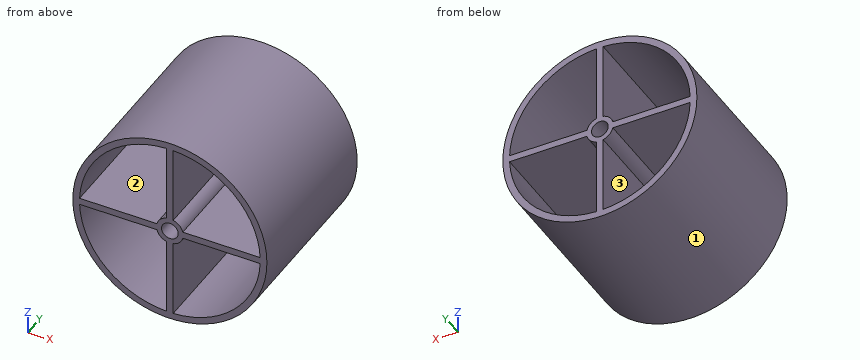
Autodesk Inventor part; units mm, degrees
ref_plane "YZ Plane" through (0, 0, 0) normal (1, 0, 0) x (0, 1, 0)
ref_plane "XZ Plane" through (0, 0, 0) normal (0, 1, 0) x (-1, 0, 0)
ref_plane "XY Plane" through (0, 0, 0) normal (0, 0, 1) x (1, 0, 0)
sketch "Boceto1" plane through (0, 0, 0) normal (0, 1, 0) x (-1, 0, 0)
  circle A0 centre (0, 0) radius 29
  dimension "d0" = 58
extrude "Extrusión1" add sketch "Boceto1" along normal blind 50
shell "Vaciado1" thickness 2 removed faces 2 at (2.104, 0, -7.1206) at (2.104, 50, -7.1206)
sketch "Boceto2" plane through (0, 0, 0) normal (0, -1, 0) x (1, 0, 0)
  line L0 (1, 28.5) -> (-1, 28.5)
  line L1 (-1, -28.5) -> (1, -28.5)
  line L2 (-28.5, 1) -> (-28.5, -1)
  line L3 (28.5, -1) -> (28.5, 1)
  line L4 (-19.4454, 20.8597) -> (-20.8597, 19.4454)
  line L5 (19.4454, -20.8597) -> (20.8597, -19.4454)
  line L6 (-64.7852, 95.7171) -> (-23.0659, 56.8262) construction
  line L7 (-20.8597, -19.4454) -> (-19.4454, -20.8597)
  line L8 (20.8597, 19.4454) -> (19.4454, 20.8597)
  arc A0 (-1, 3.873) -> (-2.0315, 3.4457) centre (0, 0) ccw
  line L9 (-1, 28.5) -> (-1, 3.873)
  line L10 (-3.873, 1) -> (-28.5, 1)
  line L11 (-28.5, -1) -> (-3.873, -1)
  line L12 (3.873, -1) -> (28.5, -1)
  line L13 (28.5, 1) -> (3.873, 1)
  line L14 (-1, -3.873) -> (-1, -28.5)
  line L15 (1, -28.5) -> (1, -3.873)
  line L16 (1, 3.873) -> (1, 28.5)
  arc A1 (3.873, 1) -> (1, 3.873) centre (0, 0) ccw
  arc A2 (1, -3.873) -> (3.873, -1) centre (0, 0) ccw
  arc A3 (1, -3.873) -> (3.873, -1) centre (0, 0) ccw
  arc A4 (-3.873, -1) -> (-1, -3.873) centre (0, 0) ccw
  arc A5 (-3.873, -1) -> (-1, -3.873) centre (0, 0) ccw
  arc A6 (-3.4457, 2.0315) -> (-3.873, 1) centre (0, 0) ccw
  arc A7 (3.873, 1) -> (1, 3.873) centre (0, 0) ccw
  arc A8 (-1, 3.873) -> (-3.873, 1) centre (0, 0) ccw
  circle A9 centre (0, 0) radius 2.5
  dimension "d4" = 2
  dimension "d5" = 57
  dimension "d6" = 57
  dimension "d7" = 2
  dimension "d12" = 2
  dimension "d13" = 57
  dimension "d14" = 57
  dimension "d15" = 2
  dimension "d17" = 5
extrude "Extrusión2" add sketch "Boceto2" against normal blind 50
properties part number "Tambor"
Read the model definition and answer for the solid it produces. Units are mm, in the model's axes. Face numbers are marked on the shaded views. Give positions to 0.01 mm unless a question says otherwise; leave off trailing zeros. Write each loop counter-clockwise with the first axis right and the second up, starting at its lowest first coordinate (ties: lowest second). Pieces come first, ordered by that corner, then holes. Notation, with made-up numbers: (17, 66) - (76, 66) arc R15 ccw to (76, 82) - close; hole circle Ø9 at (-11, -1). An arc over 180 degrees is marked (long way). Return JSON: item names as keys, results as strings.
Q1. A cutting plane is placed at C-C, the plane y = 41. Determine the outline of the cut face in (x, z), and give its area (3 significant figures).
Reply:
{"outline": "circle Ø58 at (0, 0); hole (-26.98, -1) arc R27 ccw to (-1, -26.98) - (-1, -3.87) arc R4 cw to (-3.87, -1) - close; hole (-26.98, 1) - (-3.87, 1) arc R4 cw to (-3.45, 2.03) arc R4 cw to (-2.03, 3.45) arc R4 cw to (-1, 3.87) - (-1, 26.98) arc R27 ccw to start; hole circle Ø5 at (0, 0); hole (1, -26.98) arc R27 ccw to (26.98, -1) - (3.87, -1) arc R4 cw to (1, -3.87) - close; hole (1, 3.87) arc R4 cw to (3.87, 1) - (26.98, 1) arc R27 ccw to (1, 26.98) - close", "area": "567 mm²"}
Q2. A cutting plane is placed at A-A, the plane z = 0. Determine the outline of the cut face in (x, y).
Reply:
{"outline": "(-29, 0) - (-2.5, 0) - (-2.5, 50) - (-29, 50) - close; (2.5, 0) - (29, 0) - (29, 50) - (2.5, 50) - close"}
Q3. A cutting plane is placed at B-B, the plane x = 0. Determine the outline of the cut face in (y, z).
Reply:
{"outline": "(0, -29) - (50, -29) - (50, -2.5) - (0, -2.5) - close; (0, 2.5) - (50, 2.5) - (50, 29) - (0, 29) - close"}
Q4. Consider line 1 along Z through (x, y) = (0, 25); line 2 along X through (y, z) = (21, 11); line 3 along X through (y, z) = (38, -14.5). Determine where each line is inside the solid, lowest interval first. Write a range as [from, to].
Reply:
{"line 1": "[-29, -2.5], [2.5, 29]", "line 2": "[-26.83, -24.66], [-1, 1], [24.66, 26.83]", "line 3": "[-25.11, -22.78], [-1, 1], [22.78, 25.11]"}
Q5. For a pull along Z with two mould halves and no side action, classify the marked faces 1, 2 and 3 as released by +Z, released by -Z, zero draft, split by the parting line, or undercut.
Reply:
{"face 1": "split by the parting line", "face 2": "undercut", "face 3": "undercut"}
Q6. A cutting plane is placed at D-D, the plane z = 13. Determine the outline of the cut face in (x, y), and give its area (3 significant figures).
Reply:
{"outline": "(-25.92, 0) - (-23.66, 0) - (-23.66, 50) - (-25.92, 50) - close; (-1, 0) - (1, 0) - (1, 50) - (-1, 50) - close; (23.66, 0) - (25.92, 0) - (25.92, 50) - (23.66, 50) - close", "area": "326 mm²"}
Q7. Given P1, Ø11.5, axis at x = 12.5, y = 24, coming from the -Z side; P2, Ø12, axis at x = -10.5, z = -20.5, coming from the -Y side; P3, Ø1, axis at y = 19.5, z = -22.5, coming from the -X side; P4, Ø12, axis at x = 19.5, y = 13.5, coming from the +Z side, each flat-ended and moving along its own axis, determine where each tip first touches the part or whether it passes through.
Reply:
{"P1": "z = -28.2", "P2": "y = 0", "P3": "x = -18.89", "P4": "z = 25.67"}
